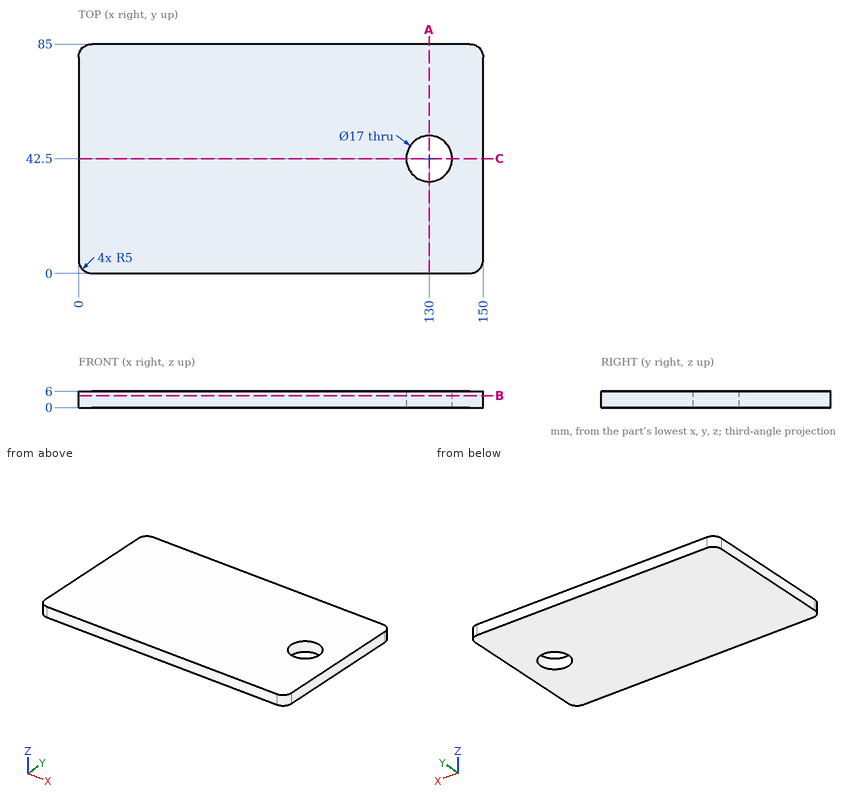
Job drawing, mm, ordinate dimensions from the low corner. One solid piece. Coordinates: 2 decimals unless noted, no trailing zeros. Order: outer loops, then holes, each group sorted by start corner. A loop starts at its lowest first (then second) coordinate and runs counter-clockwise, first axis right, second up. Notation, with made-up numbers: (38.25, 11) -> (70.25, 11) arc R28 cw to (70.25, 33) -> close; hole circle Ø11 at (41.5, 18.5). An arc over 180 degrees is marked (long way). Answer in a Markdown table with one row per item. Add a question column.
Q1. Band-saw the part on B-B, the plane z = 4.45. List the corners of the cut face in (x, y), then the cut area to 3 significant figures.
Q2. Band-saw the part on A-A, the plane x = 130. List the corners of the cut face in (y, z), then the cut area to 3 significant figures.
Q3. Drop a flat-ended pin along its axis: pin 1 (1.5 mm diameter, centred on y = 9.5, z = 4, fed in from -X). Give the stop position or say it passes through.
Q4. Band-saw the part on C-C, the plane y = 42.5. List the corners of the cut face in (x, z), then the cut area to 3 significant figures.
Q5. Wall check: line 1 along Y through (x, z) = (130, 4.25). Give the ranges that are in metal, low to high. Write a range as [from, to].
Answers follow:
| question | item | result |
|---|---|---|
| 1 | outline | (0, 5) arc R5 ccw to (5, 0) -> (145, 0) arc R5 ccw to (150, 5) -> (150, 80) arc R5 ccw to (145, 85) -> (5, 85) arc R5 ccw to (0, 80) -> close; hole circle Ø17 at (130, 42.5) |
| 1 | area | 12,500 mm^2 |
| 2 | outline | (0, 0) -> (34, 0) -> (34, 6) -> (0, 6) -> close; (51, 0) -> (85, 0) -> (85, 6) -> (51, 6) -> close |
| 2 | area | 408 mm^2 |
| 3 | pin 1 | x = 0 |
| 4 | outline | (0, 0) -> (121.5, 0) -> (121.5, 6) -> (0, 6) -> close; (138.5, 0) -> (150, 0) -> (150, 6) -> (138.5, 6) -> close |
| 4 | area | 798 mm^2 |
| 5 | line 1 | [0, 34], [51, 85] |
